The model under review builds one solid part; all positions refer to its coordinate system, in mm. A direction names the side the tool comes from. Coordinates: 2 decimals unless noted, no trailing zeros. Order: outer loops, then holes, each group sorted by start corner. A loop starts at its lowest first (then second) coordinate and runs counter-clockwise, first axis right, second up. Notation, with made-up numbers: M 29.5,-3.5 L 70.5,-3.5 A28 cw 70.5,25.5 Z; hole C 85.5,-16.5 d9. An arc over 180 degrees is marked long. Answer in a Markdown table with one row per item.
from build123d import *

# Parameters (mm, degrees)
F1_DEPTH = 15.875
F3_DEPTH = 12.7
F4_R     = 1.5875
F5_DEPTH = 17.9003632286


with BuildPart() as f1:
    # F0 (on Top) → F1 (new body)
    with BuildSketch(Plane.XY):
        with BuildLine():
            Line((0, 42.8625), (0, 0))
            Line((0, 0), (15.875, 0))
            Line((15.875, 0), (15.875, 42.8625))
            ThreePointArc((15.875, 42.8625), (7.9375, 50.8), (0, 42.8625))
        make_face()
    extrude(amount=F1_DEPTH)

    # F2 (on face) → F3 (cut)
    with BuildSketch(Plane.XY.offset(15.875)):
        with BuildLine():
            Line((2.38125, 42.8625), (2.38125, 22.225))
            ThreePointArc((2.38125, 22.225), (7.9375, 16.66875), (13.49375, 22.225))
            Line((13.49375, 22.225), (13.49375, 42.8625))
            ThreePointArc((13.49375, 42.8625), (7.9375, 48.41875), (2.38125, 42.8625))
        make_face()
    extrude(amount=-F3_DEPTH, mode=Mode.SUBTRACT)

    # F4 (on face) → F5 (cut, up to face)
    with BuildSketch(Plane.XZ):
        with Locations((7.9375, 7.9375)):
            Circle(F4_R)
    extrude(amount=-F5_DEPTH, mode=Mode.SUBTRACT)


solid = f1.part
(1) To check wall thickness, follow line 1 (X direction, y = 23, z = 8.75) (3 decimals); line 2 (X direction, y = 6, z = 8) (3 decimals); line 3 (Y direction, x = 10, z = 11.75). State the ranges of each line that lie inside material, in increasing order. Write a range as [from, to].
Report:
| item | result |
|---|---|
| line 1 | [0, 2.381], [13.494, 15.875] |
| line 2 | [0, 6.351], [9.524, 15.875] |
| line 3 | [0, 17.07], [48.02, 50.53] |
(2) Machinability: for faces 4 (the flat face through (15.875, 21, 8)), 5 (the flat face through (13.494, 32, 10)), which of the approach directions +Z, -Z, +X, -X, +Y, -Y give a long, thin tool a straight path to every point of the face, cutting with its end or side? Answer none if there is none.
Report:
| item | result |
|---|---|
| face 4 | +Z, -Z, +X, +Y, -Y |
| face 5 | +Z |
(3) Insertion check: P1, Ø6, axis at x = 11.5, z = 3, coming from the +Y side; P2, Ø3, axis at x = 10.5, z = 13, coming from the +Y side; P3, Ø2, axis at x = 4.5, z = 4.5, coming from the +Y side. Each pin has a flat end and moves straight along its axis. Give the tip position at first contact, or say it passes through.
Report:
| item | result |
|---|---|
| P1 | y = 50.78 |
| P2 | y = 50.73 |
| P3 | y = 50.42 |
(4) Take a section at A-A (z = 11.25). Write out the cut boundary in (x, y) (1 decimal), then the cut area to 3 significant figures.
Report:
| item | result |
|---|---|
| outline | M 0,0 L 15.9,0 L 15.9,42.9 A7.9 ccw 0,42.9 Z; hole M 2.4,22.2 A5.6 ccw 13.5,22.2 L 13.5,42.9 A5.6 ccw 2.4,42.9 Z |
| area | 453 mm^2 |
(5) Take a section at C-C (y = 24). Write out the cut boundary in (x, z) (3 decimals).
Report:
| item | result |
|---|---|
| outline | M 0,0 L 15.875,0 L 15.875,15.875 L 13.494,15.875 L 13.494,3.175 L 2.381,3.175 L 2.381,15.875 L 0,15.875 Z |
(6) Take a section at B-B (x = 7.5). Write out the cut boundary in (y, z) (1 decimal).
Report:
| item | result |
|---|---|
| outline | M 0,0 L 50.8,0 L 50.8,15.9 L 48.4,15.9 L 48.4,3.2 L 16.7,3.2 L 16.7,6.4 L 0,6.4 Z; M 0,9.5 L 16.7,9.5 L 16.7,15.9 L 0,15.9 Z |
(7) The part is to be moulded in two halves that separate along X. For faces 1 (the flat face through (6, 0, 8)), 2 (the cylindrical face through (9.452, 8.335, 8.414)), 3 (the flat face through (0, 22, 8)), say which applies: +X half, -X half, draft (parallel to the pull), parting line (faces both ways), or undercut.
Report:
| item | result |
|---|---|
| face 1 | draft |
| face 2 | undercut |
| face 3 | -X half |
(8) Take a section at D-D (x = 4). Write out the cut boundary in (y, z) (3 decimals), then the cut area to 3 significant figures.
Report:
| item | result |
|---|---|
| outline | M 0,0 L 49.755,0 L 49.755,15.875 L 46.783,15.875 L 46.783,3.175 L 18.305,3.175 L 18.305,15.875 L 0,15.875 Z |
| area | 428 mm^2 |
